Source: CAD feature listing. Evaluate the final solid. Frame: model axes, mm. Face numbers are marked on the shaded views. A direction names the side the tool comes from. Coordinates: 2 decimals unless noted, no trailing zeros. Order: outer loops, then holes, each group sorted by start corner. A loop starts at its lowest first (then second) coordinate and runs counter-clockwise, first axis right, second up. Notation, with made-up numbers: (47, -5.5) - (68, -5.5) arc R17 ccw to (68, 13.5) - close; hole circle Ø7 at (-8.75, 13.25). An arc over 180 degrees is marked (long way). One line per question, with ' | ' between items.
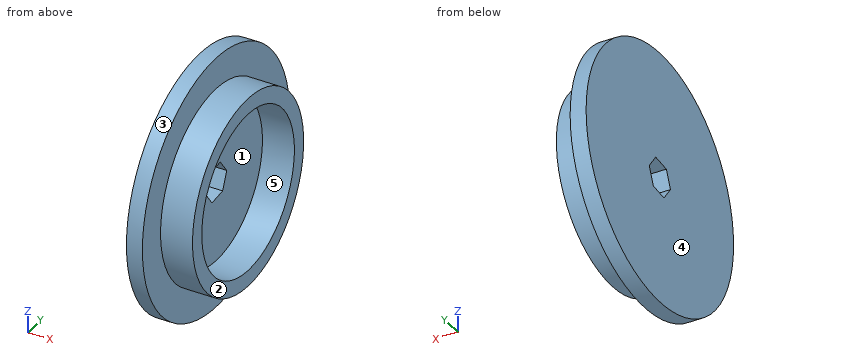
Autodesk Inventor part; units mm, degrees
ref_plane "YZ Plane" through (0, 0, 0) normal (1, 0, 0) x (0, 1, 0)
ref_plane "XZ Plane" through (0, 0, 0) normal (0, 1, 0) x (-1, 0, 0)
ref_plane "XY Plane" through (0, 0, 0) normal (0, 0, 1) x (1, 0, 0)
sketch "Sketch1" plane through (0, 0, 0) normal (1, 0, 0) x (0, 1, 0)
  circle A0 centre (0, 0) radius 50.546
  dimension "d0" = 101.092
extrude "Extrusion1" add sketch "Sketch1" along normal blind 6.35
sketch "Sketch2" plane through (6.35, 0, 0) normal (1, 0, 0) x (0, 0, -1)
  circle A0 centre (0, 0) radius 38.1
  circle A1 centre (0, 0) radius 31.75
  dimension "d3" = 76.2
  dimension "d4" = 6.35
extrude "Extrusion2" add sketch "Sketch2" along normal blind 12.7
sketch "Sketch3" plane through (6.35, 0, 0) normal (1, 0, 0) x (0, 0, -1)
  line L0 (-6.7678, 2.8213) -> (-0.9406, 7.2718)
  line L1 (-0.9406, 7.2718) -> (5.8273, 4.4504)
  line L2 (5.8273, 4.4504) -> (6.7678, -2.8213)
  line L3 (6.7678, -2.8213) -> (0.9406, -7.2718)
  line L4 (0.9406, -7.2718) -> (-5.8273, -4.4504)
  line L5 (-5.8273, -4.4504) -> (-6.7678, 2.8213)
  point P0 (0, 0)
  point P1 (0, 0)
  dimension "d7" = 12.7
extrude "Extrusion3" cut sketch "Sketch3" against normal blind 12.7
properties part number "wheel hub"
(1) Pull-direction query (Y, two-part tool) for the marked faces 3, 4 and 5; classes: pulls with the +Y half, pulls with the -Y half, needs draft (parallel to the pull), parting line crosses it, or undercut.
Taken from the geometry:
face 3: parting line crosses it | face 4: needs draft | face 5: undercut
(2) Material intervals for L1, parallel to Y at x = 15.5, z = 0; L2, parallel to X at y = -26, z = -41.5; L3, parallel to Y at x = 10.25, z = 26, sorted ascending. Write a range as from..to.
Taken from the geometry:
L1: y = -38.1..-31.75, 31.75..38.1 | L2: x = 0..6.35 | L3: y = -27.85..-18.22, 18.22..27.85
(3) Cut plane A-A (x = 3.25). Return the cut outline in (y, z).
Taken from the geometry:
outline: circle Ø101.09 at (0, 0); hole (-7.27, -0.94) - (-2.82, -6.77) - (4.45, -5.83) - (7.27, 0.94) - (2.82, 6.77) - (-4.45, 5.83) - close
(4) Set-up query: the marked faces 1 and 2. Return all of +Z, -Z, +X, -X, +Y, -Y with unobstructed straight access to the full face (end or side cutting, diameter ignored); none if empty.
Taken from the geometry:
face 1: +X | face 2: +Z, -Z, +X, +Y, -Y
(5) Pin query (flat end, axial travel): P1, Ø6, axis at x = 13.5, y = -6.5, coming from the -Z side; P2, Ø6, axis at x = 9.5, z = 12, coming from the -Y side; P3, Ø4, axis at x = 9, y = -4, coming from the +Z side; P4, Ø2, axis at x = 3, z = 1, coming from the +Y side. Return the tip coordinate at first contact, or that it passes through.
Taken from the geometry:
P1: stops at z = -37.94 | P2: stops at y = -37.02 | P3: stops at z = 38.05 | P4: stops at y = 50.55
(6) Cut plane D-D (y = 19.5). Return the cut outline in (x, z).
Taken from the geometry:
outline: (0, -46.63) - (6.35, -46.63) - (6.35, -32.73) - (19.05, -32.73) - (19.05, -25.06) - (6.35, -25.06) - (6.35, 25.06) - (19.05, 25.06) - (19.05, 32.73) - (6.35, 32.73) - (6.35, 46.63) - (0, 46.63) - close
(7) Cut plane B-B (z = -11.5). Return the cut outline in (x, y).
Taken from the geometry:
outline: (0, -49.22) - (6.35, -49.22) - (6.35, -36.32) - (19.05, -36.32) - (19.05, -29.59) - (6.35, -29.59) - (6.35, 29.59) - (19.05, 29.59) - (19.05, 36.32) - (6.35, 36.32) - (6.35, 49.22) - (0, 49.22) - close
(8) Cut plane C-C (y = 0). Return the cut outline in (x, z).
Taken from the geometry:
outline: (0, -50.55) - (6.35, -50.55) - (6.35, -38.1) - (19.05, -38.1) - (19.05, -31.75) - (6.35, -31.75) - (6.35, -6.4) - (0, -6.4) - close; (0, 6.4) - (6.35, 6.4) - (6.35, 31.75) - (19.05, 31.75) - (19.05, 38.1) - (6.35, 38.1) - (6.35, 50.55) - (0, 50.55) - close
